Geometry check sheet. Reference: drawing and pictorial views, mm from the part's lowest x, y, z. Coordinates: 2 decimals unless noted, no trailing zeros. Write each loop counter-clockwise with the first axis right and the second up, starting at its lowest first coordinate (ties: lowest second). Pieces come first, ordered by that corner, then holes. Notation, with made-up numbers: (11, 72) -> (53, 72) arc R19 cw to (53, 97) -> close; hole circle Ø9 at (86, 18). An arc over 180 degrees is marked (long way). Put each result on its own line as item: value.
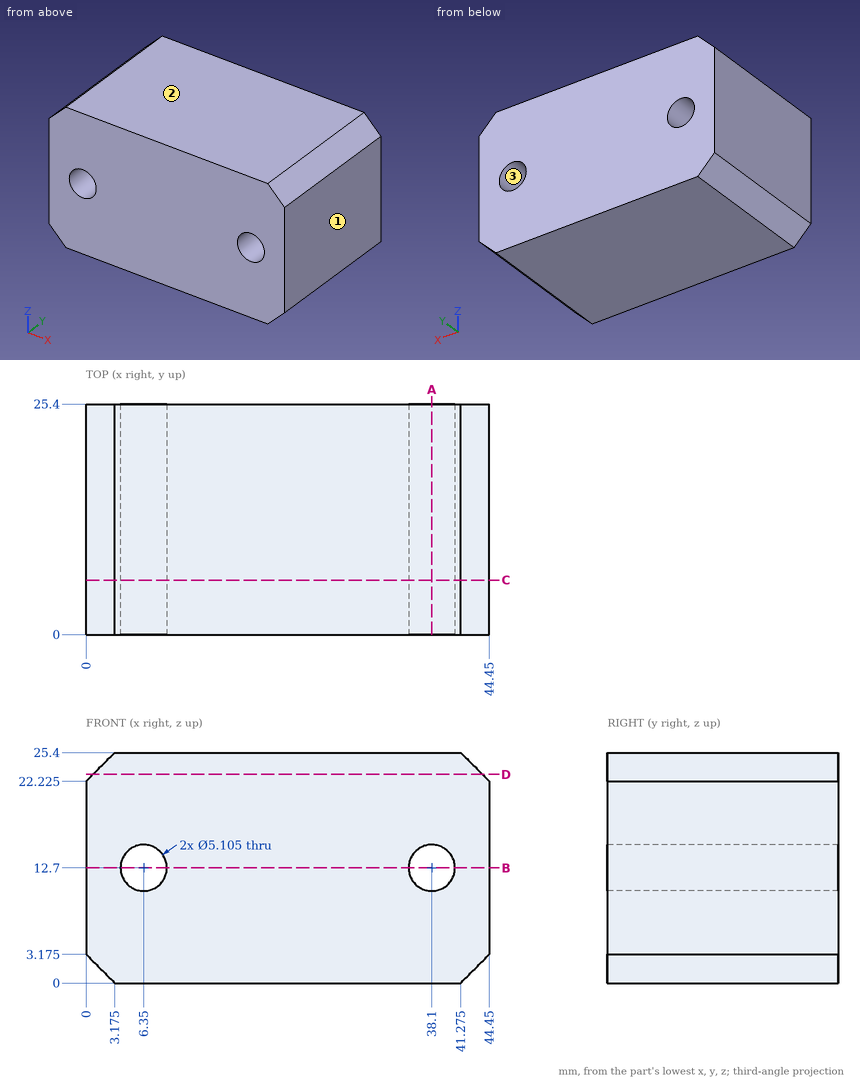
Q1. Cross-section at D-D (z = 23). Record the cut outline in (x, y) (1 decimal).
Recorded:
outline: (0.8, 0) -> (43.7, 0) -> (43.7, 25.4) -> (0.8, 25.4) -> close
Q2. Material ranges on line 1 along Z through (x, y) = (6.35, 7); line 2 along X through (y, z) = (10.75, 14); line 3 along X through (y, z) = (22, 12.25), recorded low to high.
Recorded:
line 1: z = 0 to 10.15, 15.25 to 25.4
line 2: x = 0 to 4.15, 8.55 to 35.9, 40.3 to 44.45
line 3: x = 0 to 3.84, 8.86 to 35.59, 40.61 to 44.45
Q3. Mould release check, pull along X, two halves, no side actions. Record for the marked faces 1, 2 and 3: released by +X, released by -X, zero draft, split by the parting line, or undercut.
Recorded:
face 1: released by +X
face 2: zero draft
face 3: undercut
Q4. Cross-section at A-A (x = 38.1). Record the cut outline in (y, z).
Recorded:
outline: (0, 0) -> (25.4, 0) -> (25.4, 10.15) -> (0, 10.15) -> close; (0, 15.25) -> (25.4, 15.25) -> (25.4, 25.4) -> (0, 25.4) -> close
Q5. Cross-section at B-B (z = 12.7). Record the cut outline in (x, y).
Recorded:
outline: (0, 0) -> (3.8, 0) -> (3.8, 25.4) -> (0, 25.4) -> close; (8.9, 0) -> (35.55, 0) -> (35.55, 25.4) -> (8.9, 25.4) -> close; (40.65, 0) -> (44.45, 0) -> (44.45, 25.4) -> (40.65, 25.4) -> close
Q6. Cross-section at C-C (y = 6). State how many separate pieces and enclosed holes the cut face has, plus the area to 3 significant figures.
Recorded:
separate pieces: 1
enclosed holes: 2
area: 1,070 mm2
